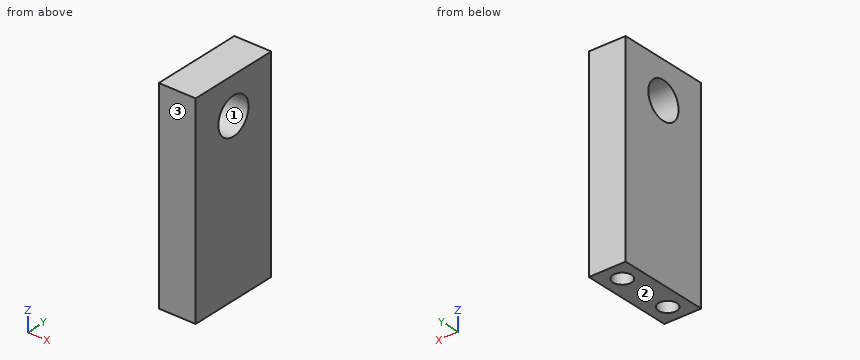
```python
from build123d import *

# Parameters (mm, degrees)
SKETCH1_W           = 12.7
SKETCH1_H           = 31.75
SKETCH1_R           = 3.175
BOSS_EXTRUDE1_DEPTH = 69.85
SKETCH2_R           = 3.175
BOSS_EXTRUDE2_DEPTH = 50.8
SKETCH3_R           = 6.35
CUT_EXTRUDE1_DEPTH  = 13.7


with BuildPart() as part:
    # Sketch1 → Boss-Extrude1 (new body)
    with BuildSketch(Plane.XY):
        Rectangle(SKETCH1_W, SKETCH1_H)
        with Locations((0, 9.525)):
            Circle(SKETCH1_R, mode=Mode.SUBTRACT)
        with Locations((0, -9.525)):
            Circle(SKETCH1_R, mode=Mode.SUBTRACT)
    extrude(amount=BOSS_EXTRUDE1_DEPTH)

    # Sketch2 → Boss-Extrude2 (add)
    with BuildSketch(Plane.XY.offset(69.85)):
        with Locations((0, -9.525)):
            Circle(SKETCH2_R)
        with Locations((0, 9.525)):
            Circle(SKETCH2_R)
    extrude(amount=-BOSS_EXTRUDE2_DEPTH)

    # Sketch3 → Cut-Extrude1 (cut, through all)
    with BuildSketch(Plane(origin=(6.35, 0, 0), x_dir=(0, 0, -1), z_dir=(1, 0, 0))):
        with Locations((-57.15, 0)):
            Circle(SKETCH3_R)
    extrude(amount=-CUT_EXTRUDE1_DEPTH, mode=Mode.SUBTRACT)


solid = part.part
```
Geometry: final body of the model. Coordinates: model frame, mm. Face numbers are marked on the shaded views. Round coordinates to 2 decimals unless told otherwise and drop trailing zeros. Order: outer loops, then holes, each group sorted by start corner. A loop starts at its lowest first (then second) coordinate and runs counter-clockwise, first axis right, second up. Notation, with made-up numbers: (33.25, 79) - (46.25, 79) arc R27 ccw to (46.25, 110) - close; hole circle Ø4 at (32.25, 45.5). An arc over 180 degrees is marked (long way). Use CSV: the item, a comma, the result in double quotes. Start each with the question number.
Q1. Mould query, pull axis Y, two halves, no side actions, for the marked faces 1, 2 and 3. Classes: +Y half, -Y half, draft (parallel to the pull), parting line (faces both ways), or undercut.
Q2. First-contact query: pin 1 (5 mm diameter, centred on x = 0, y = -9.525, fed in from -Z); pin 2 (6 mm diameter, centred on x = -1, y = -7.5, fed in from -Z). Flat tips, straight axial feed; report the tip coordinate or a pass-through.
Q3. Material intervals for line 1 along Y through (x, z) = (0, 10.25) (3 decimals); line 2 along Y through (x, z) = (-0.5, 57.15) (3 decimals); line 3 along X through (y, z) = (9.5, 14.5), sorted ascending. Write a range as from..to.
Q4. Section query A-A (y = 0). Return loops of the section in (x, z).
Q5. Section query C-C (z = 57.15). Return loops of the section in (x, y) (3 decimals), and give its area (3 significant figures).
Q6. Section query B-B (x = 0). Return loops of the section in (y, z) (3 decimals), and give its area (3 significant figures).
Q7. Section query D-D (y = -12). Return loops of the section in (x, z).
Result set:
1,face 1,"undercut"
1,face 2,"draft"
1,face 3,"-Y half"
2,pin 1,"stops at z = 19.05"
2,pin 2,"stops at z = 0"
3,line 1,"y = -15.875..-12.7, -6.35..6.35, 12.7..15.875"
3,line 2,"y = -15.875..-6.35, 6.35..15.875"
3,line 3,"x = -6.35..-3.17, 3.17..6.35"
4,outline,"(-6.35, 0) - (6.35, 0) - (6.35, 50.8) - (-6.35, 50.8) - close; (-6.35, 63.5) - (6.35, 63.5) - (6.35, 69.85) - (-6.35, 69.85) - close"
5,outline,"(-6.35, -15.875) - (6.35, -15.875) - (6.35, -6.35) - (-6.35, -6.35) - close; (-6.35, 6.35) - (6.35, 6.35) - (6.35, 15.875) - (-6.35, 15.875) - close"
5,area,"242 mm2"
6,outline,"(-15.875, 0) - (-12.7, 0) - (-12.7, 19.05) - (-6.35, 19.05) - (-6.35, 0) - (6.35, 0) - (6.35, 19.05) - (12.7, 19.05) - (12.7, 0) - (15.875, 0) - (15.875, 69.85) - (-15.875, 69.85) - close; hole circle Ø12.7 at (0, 57.15)"
6,area,"1,850 mm2"
7,outline,"(-6.35, 0) - (-1.99, 0) - (-1.99, 19.05) - (1.99, 19.05) - (1.99, 0) - (6.35, 0) - (6.35, 69.85) - (-6.35, 69.85) - close"
